from build123d import *

# Parameters (mm, degrees)
SKETCH1_W      = 30
SKETCH1_H      = 15
SKETCH1_H_2    = 5
EXTRUDE1_DEPTH = 8
EXTRUDE2_START = 5
SKETCH2_R      = 2
SKETCH2_W      = 30.8
SKETCH2_H      = 12
SKETCH2_W_2    = 22.8
SKETCH2_H_2    = 8
EXTRUDE2_DEPTH = 20
EXTRUDE3_START = 6
SKETCH3_W      = 28
SKETCH3_H      = 14
EXTRUDE3_DEPTH = 2
SKETCH3_3_W    = 4
SKETCH3_3_H    = 17
EXTRUDE4_DEPTH = 4
EXTRUDE5_START = -15
SKETCH2_3_W    = 22.8
SKETCH2_3_H    = 8
EXTRUDE5_DEPTH = 3
EXTRUDE6_START = -18
EXTRUDE6_DEPTH = 23


with BuildPart() as part:
    # Sketch1 → Extrude1 (new, symmetric)
    with BuildSketch(Plane.XY):
        Polygon((-15, 0), (-15, 5), (-23, 5), (-23, -1), (-18, -1), (-18, -18), (18, -18), (18, -1), (23, -1), (23, 5), (15, 5), (15, 0), (15, -15), (-15, -15), align=None)
        with Locations((0, -7.5)):
            Rectangle(SKETCH1_W, SKETCH1_H)
        with Locations((0, 2.5)):
            Rectangle(SKETCH1_W, SKETCH1_H_2)
    extrude(amount=EXTRUDE1_DEPTH, both=True)

    # Sketch2 → Extrude2 (cut)
    with BuildSketch(Plane(origin=(0, 0, 0), x_dir=(1, 0, 0), z_dir=(0, 1, 0)).offset(EXTRUDE2_START)):
        Polygon((-23, -8), (-23, -3.1), (-18.1, -8), align=None)
        with Locations(Location((-18.1, 0, 0), (0, 0, 272.865983983))):
            Circle(SKETCH2_R)
        Polygon((-23, 8), (-18.1, 8), (-23, 3.1), align=None)
        Rectangle(SKETCH2_W, SKETCH2_H)
        Rectangle(SKETCH2_W_2, SKETCH2_H_2, mode=Mode.SUBTRACT)
        Rectangle(SKETCH2_W_2, SKETCH2_H_2)
        Polygon((23, 3.1), (23, 8), (18.1, 8), align=None)
        with Locations(Location((18.1, 0, 0), (0, 0, 267.134016017))):
            Circle(SKETCH2_R)
        Polygon((18.1, -8), (23, -8), (23, -3.1), align=None)
    extrude(amount=-EXTRUDE2_DEPTH, mode=Mode.SUBTRACT)

    # Sketch3 (on Front Plane) → Extrude3 (cut)
    with BuildSketch(Plane.XY.offset(EXTRUDE3_START)):
        with Locations((0, -7)):
            Rectangle(SKETCH3_W, SKETCH3_H)
    extrude(amount=EXTRUDE3_DEPTH, mode=Mode.SUBTRACT)

    # Sketch3<3> → Extrude4 (cut, symmetric)
    with BuildSketch(Plane.XY):
        with Locations((-16, -9.5)):
            Rectangle(SKETCH3_3_W, SKETCH3_3_H)
        with Locations((16, -9.5)):
            Rectangle(SKETCH3_3_W, SKETCH3_3_H)
    extrude(amount=EXTRUDE4_DEPTH, both=True, mode=Mode.SUBTRACT)

    # Sketch2<3> → Extrude5 (cut)
    with BuildSketch(Plane(origin=(0, 0, 0), x_dir=(1, 0, 0), z_dir=(0, 1, 0)).offset(EXTRUDE5_START)):
        Rectangle(SKETCH2_3_W, SKETCH2_3_H)
    extrude(amount=-EXTRUDE5_DEPTH, mode=Mode.SUBTRACT)

    # Sketch4 → Extrude6 (add)
    with BuildSketch(Plane(origin=(0, 0, 0), x_dir=(1, 0, 0), z_dir=(0, 1, 0)).offset(EXTRUDE6_START)):
        with BuildLine():
            Line((10.386751346, 8), (18, 8))
            ThreePointArc((18, 8), (14.464466094, 9.464466094), (13, 13))
            Line((13, 13), (7.5, 13))
            Line((7.5, 13), (10.386751346, 8))
        make_face()
        with BuildLine():
            Line((-9, 8), (-1.386751346, 8))
            Line((-1.386751346, 8), (1.5, 13))
            Line((1.5, 13), (-4, 13))
            ThreePointArc((-4, 13), (-5.464466094, 9.464466094), (-9, 8))
        make_face()
    extrude(amount=EXTRUDE6_DEPTH)


solid = part.part
Could you check a few things on this model? Use its own coordinates, in mm. A direction names the side the tool comes from. Round coordinates to 2 decimals unless told otherwise and drop trailing zeros. Order: outer loops, then holes, each group sorted by start corner. A loop starts at its lowest first (then second) coordinate and runs counter-clockwise, first axis right, second up.
Q1. Imagine slicing it at A-A, the plane y = -11.5. List the corners of the cut face in (x, z) for me, then the cut area to 3 significant figures.
Geometry says:
outline: (-18, -8) - (-9, -8) arc R5 cw to (-4, -13) - (1.5, -13) - (-1.39, -8) - (10.39, -8) - (7.5, -13) - (13, -13) arc R5 cw to (18, -8) - (18, -4) - (15.4, -4) - (15.4, -6) - (-15.4, -6) - (-15.4, -4) - (-18, -4) - close; (-18, 4) - (-15.4, 4) - (-15.4, 6) - (-14, 6) - (-14, 8) - (-18, 8) - close; (14, 6) - (15.4, 6) - (15.4, 4) - (18, 4) - (18, 8) - (14, 8) - close
area: 160 mm2
Q2. Imagine slicing it at C-C, the plane x = -0.5. List the corners of the cut face in (y, z) for me, then the cut area to 3 significant figures.
Geometry says:
outline: (-18, -13) - (5, -13) - (5, -9.54) - (-18, -9.54) - close; (-18, -8) - (5, -8) - (5, -6) - (-15, -6) - (-15, -4) - (-18, -4) - close; (-18, 4) - (-15, 4) - (-15, 6) - (-14, 6) - (-14, 8) - (-18, 8) - close; (0, 6) - (5, 6) - (5, 8) - (0, 8) - close
area: 156 mm2
Q3. Which directions (+Z, -Z, +X, -X, +Y, -Y) give clear straight access to the entire face, cutting with the end or side of a thin tool? Please do faces 5 (the face through (-14, -6, -8)), 6 (the face through (-18, -9, -6)), 7 (the face through (0.036, -6.661, -10.465)), 8 (the face through (-15.4, 0, 0)).
Geometry says:
face 5: -Z, -X, +Y, -Y
face 6: +Z, -Z, -X, -Y
face 7: +Y, -Y
face 8: +Y
Q4. Imagine slicing it at D-D, the plane y = -14.5. List the corners of the cut face in (x, z) for me, then the cut area to 3 significant figures.
Geometry says:
outline: (-18, -8) - (-9, -8) arc R5 cw to (-4, -13) - (1.5, -13) - (-1.39, -8) - (10.39, -8) - (7.5, -13) - (13, -13) arc R5 cw to (18, -8) - (18, -4) - (15.4, -4) - (15.4, -6) - (-15.4, -6) - (-15.4, -4) - (-18, -4) - close; (-18, 4) - (-15.4, 4) - (-15.4, 6) - (15.4, 6) - (15.4, 4) - (18, 4) - (18, 8) - (-18, 8) - close
area: 216 mm2
Q5. I'm going to push flat-ended pins straight in: P1, Ø1.6, axis at y = -7.5, z = 7, coming from the +X side; P2, Ø4.5, axis at x = 18.1, z = 0, coming from the +Y side; P3, Ø1, axis at x = -10.5, y = -3.5, coming from the +Z side; P4, Ø2, axis at y = -9, z = 6, coming from the -X side. Where does each tip first touch, or does it pass through?
Geometry says:
P1: stops at x = 18
P2: stops at y = 5
P3: stops at z = -6
P4: stops at x = -18
Q6. Please list where these lines run through material, in increasing order: probe 1 along X at (y, z) = (3.2, 0); probe 2 along Z at (x, y) = (18.1, 0.3); probe 3 along X at (y, z) = (-7.5, 6.75).
Geometry says:
probe 1: x = -23 to -20.1, -16.1 to -15.4, 15.4 to 16.1, 20.1 to 23
probe 2: z = -8 to -2, 2 to 8
probe 3: x = -18 to -14, 14 to 18
Q7. Imagine slicing it at B-B, the plane z = -0.5. List the corners of the cut face in (x, y) for me, then the cut area to 3 significant figures.
Geometry says:
outline: (-23, -1) - (-20.04, -1) - (-20.04, 5) - (-23, 5) - close; (-16.16, -1) - (-15.4, -1) - (-15.4, 5) - (-16.16, 5) - close; (-14, -18) - (-11.4, -18) - (-11.4, -15) - (-14, -15) - close; (11.4, -18) - (14, -18) - (14, -15) - (11.4, -15) - close; (15.4, -1) - (16.16, -1) - (16.16, 5) - (15.4, 5) - close; (20.04, -1) - (23, -1) - (23, 5) - (20.04, 5) - close
area: 60.3 mm2
Q8. Thinking about a two-plate mould opening in Y: for faces 1 (the face through (14, -7, 7)), 2 (the face through (0, 0, 7)), 3 (the face through (-16, -9, 4)), 4 (the face through (0, 5, -7)), which applies, released by +Y, released by -Y, zero draft, split by the parting line, or undercut?
Geometry says:
face 1: undercut
face 2: undercut
face 3: zero draft
face 4: released by +Y
